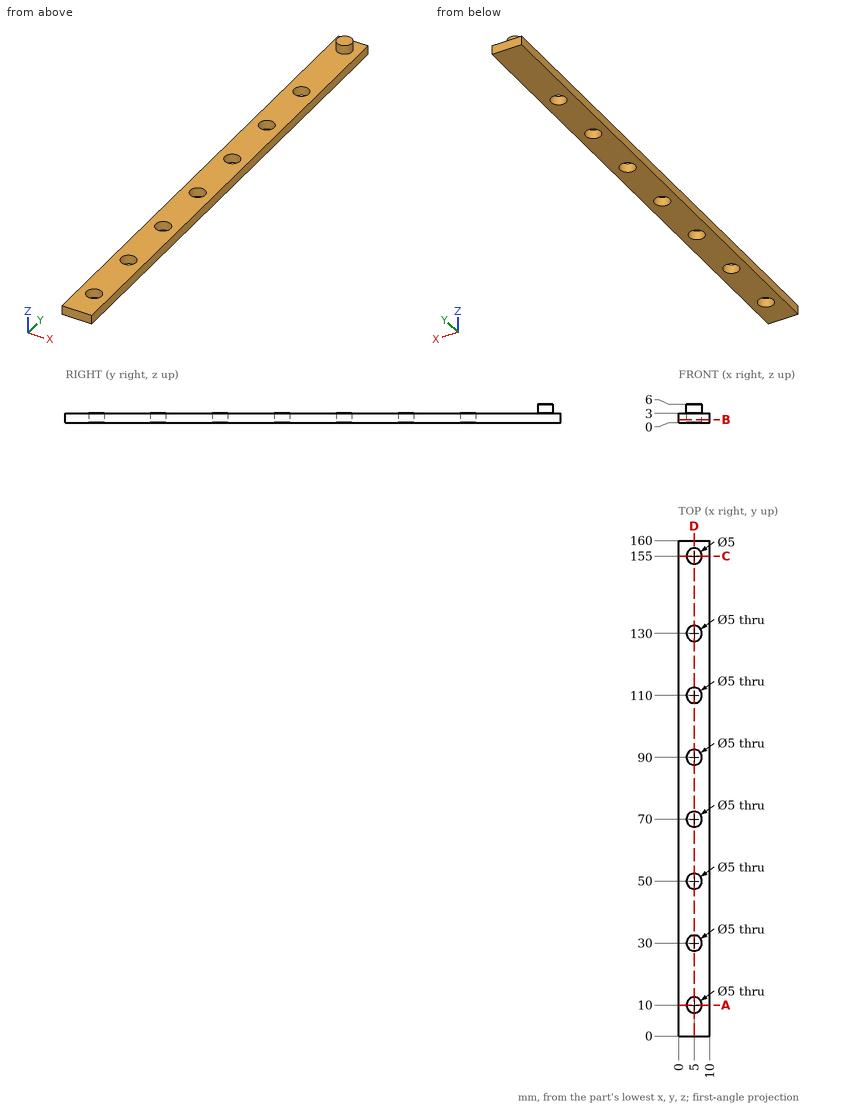
For this review, use the dimensioned drawing (mm, ordinates from the lowest corner) and the shaded views. Coordinates: 2 decimals unless noted, no trailing zeros. Loops run counter-clockwise (first coordinate to the right, second up) from the corner with the lowest first, then second, coordinate; pieces in that order, holes last. Notation, with made-up numbers: (-3, 71.25) -> (1, 71.25) arc R23 ccw to (1, 99.25) -> close; hole circle Ø10 at (-28.5, 57.25). An arc over 180 degrees is marked (long way). Write each question's results on one line, items separated by ' | '.
Q1. Add section A-A, the plane y = 10. State the section outline as (x, z) points.
Taken from the geometry:
outline: (0, 0) -> (2.5, 0) -> (2.5, 3) -> (0, 3) -> close; (7.5, 0) -> (10, 0) -> (10, 3) -> (7.5, 3) -> close
Q2. Add section B-B, the plane z = 0.95. State the section outline as (x, y) points.
Taken from the geometry:
outline: (0, 0) -> (10, 0) -> (10, 160) -> (0, 160) -> close; hole circle Ø5 at (5, 10); hole circle Ø5 at (5, 30); hole circle Ø5 at (5, 50); hole circle Ø5 at (5, 70); hole circle Ø5 at (5, 90); hole circle Ø5 at (5, 110); hole circle Ø5 at (5, 130)
Q3. Add section D-D, the plane x = 5. Count the separate pieces of the cut face and the enclosed holes in it, then the cut area to 3 significant figures.
Taken from the geometry:
separate pieces: 8 | enclosed holes: 0 | area: 390 mm²
Q4. Add section C-C, the plane y = 155. State the section outline as (x, z) points.
Taken from the geometry:
outline: (0, 0) -> (10, 0) -> (10, 3) -> (7.5, 3) -> (7.5, 6) -> (2.5, 6) -> (2.5, 3) -> (0, 3) -> close
Q5. For pin 1 Ø2 at (x, y) = (3, 87) entering from -Z; pin 2 Ø5 at (x, y) = (4, 102.5) entering from +Z, all flat-tipped, find the tip position at first contact; note any pin that passes through.
Taken from the geometry:
pin 1: z = 0 | pin 2: z = 3
Q6. To check wall thickness, follow line 1 along X through (y, z) = (130, 1.25); line 2 along Z through (x, y) = (4, 53.5); line 3 along X through (y, z) = (68, 0.6). State the ranges of each line that lie inside material, in increasing order. Write a range as [from, to].
Taken from the geometry:
line 1: [0, 2.5], [7.5, 10] | line 2: [0, 3] | line 3: [0, 3.5], [6.5, 10]
